```python
from build123d import *

# Parameters (mm, degrees)
F0_W     = 106.68
F0_H     = 157.48
F1_DEPTH = 106.68
F2_W     = 100.33
F2_H     = 151.13
F3_DEPTH = 101.6
F4_W     = 106.68
F4_H     = 1.5875
F5_DEPTH = 101.6
F6_R     = 5.08


with BuildPart() as f1:
    # F0 (on Front) → F1 (new body)
    with BuildSketch(Plane.XZ):
        with Locations((2.224307, 32.226964)):
            Rectangle(F0_W, F0_H)
    extrude(amount=F1_DEPTH)

    # F2 (on face) → F3 (cut)
    with BuildSketch(Plane.XZ.offset(106.68)):
        with Locations((2.224307, 32.226964)):
            Rectangle(F2_W, F2_H)
    extrude(amount=-F3_DEPTH, mode=Mode.SUBTRACT)

    # F4 (on face) → F5 (join)
    with BuildSketch(Plane.XZ.offset(106.68)):
        with Locations((2.224307, 56.198214)):
            Rectangle(F4_W, F4_H)
        with Locations((2.224307, 57.785714)):
            Rectangle(F4_W, F4_H)
        with Locations((2.224307, 6.985714)):
            Rectangle(F4_W, F4_H)
        with Locations((2.224307, 5.398214)):
            Rectangle(F4_W, F4_H)
    extrude(amount=-F5_DEPTH)

    # F6
    f6_edges = [f1.edges().sort_by_distance(p)[0] for p in [
        (55.564307, -53.34, 110.966964),
        (-51.115693, -53.34, 110.966964),
        (55.564307, -53.34, -46.513036),
        (-51.115693, -53.34, -46.513036),
        (-51.115693, 0, 32.226964),
        (2.224307, 0, 110.966964),
        (55.564307, 0, 32.226964),
        (2.224307, 0, -46.513036),
    ]]
    fillet(f6_edges, radius=F6_R)


solid = f1.part
```
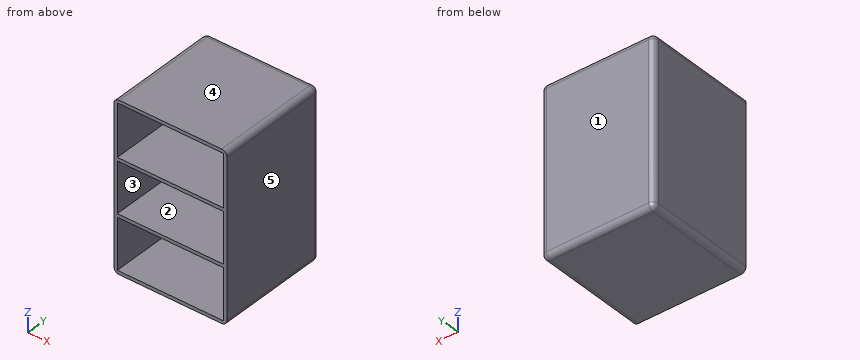
Here's how the part is built. I have some questions about the finished solid (model axes, mm). Face numbers are marked on the shaded views. A direction names the side the tool comes from. Round coordinates to 2 decimals unless told otherwise and drop trailing zeros. Order: outer loops, then holes, each group sorted by start corner. A loop starts at its lowest first (then second) coordinate and runs counter-clockwise, first axis right, second up. Notation, with made-up numbers: (-9.75, 44) -> (9.25, 44) arc R24 cw to (9.25, 78) -> close; hole circle Ø9 at (26.5, 30.5). An arc over 180 degrees is marked (long way). Use a Markdown table: item, result. Add a question column.
(1) Suppose I cut it at B-B, the plane y = -97. Please give me the cut outline in (x, z).
(2) Suppose I cut it at A-A, the plane z = 61. Please give me the cut outline in (x, y), and give its area (3 significant figures).
(3) For the marked faces 1 and 2, which set-ups out of +Z, -Z, +X, -X, +Y, -Y let a thin tool reach every point of the face, with its end or its side?
(4) For pin 1 Ø14.5 at (x, z) = (-16.5, 25) entering from -Y, with a flat end and sliding along its axis, tell me the tip position at first contact or that it passes through.
(5) Suppose I cut it at C-C, the plane x = -1. Please give me the cut outline in (y, z).
(6) If we mould it in two halves opening along X, with no side actions, what happens to the marked faces 3, 4 and 5? For each: released by +X, released by -X, zero draft, split by the parting line, or undercut.
(7) I need wall thicknesses on line 1 along Z through (x, y) = (38.5, -101); line 2 along X through (y, z) = (-80, 50); line 3 along Y through (x, z) = (-15, 89). Which ranges of each line are inside material? Lowest first, please.
Verdict:
| question | item | result |
|---|---|---|
| 1 | outline | (-51.12, -41.43) arc R5.08 ccw to (-46.04, -46.51) -> (50.48, -46.51) arc R5.08 ccw to (55.56, -41.43) -> (55.56, 105.89) arc R5.08 ccw to (50.48, 110.97) -> (-46.04, 110.97) arc R5.08 ccw to (-51.12, 105.89) -> close; hole (-47.94, -43.34) -> (52.39, -43.34) -> (52.39, 4.6) -> (-47.94, 4.6) -> close; hole (-47.94, 7.78) -> (52.39, 7.78) -> (52.39, 55.4) -> (-47.94, 55.4) -> close; hole (-47.94, 58.58) -> (52.39, 58.58) -> (52.39, 107.79) -> (-47.94, 107.79) -> close |
| 2 | outline | (-51.12, -106.68) -> (-47.94, -106.68) -> (-47.94, -5.08) -> (52.39, -5.08) -> (52.39, -106.68) -> (55.56, -106.68) -> (55.56, -5.08) arc R5.08 ccw to (50.48, 0) -> (-46.04, 0) arc R5.08 ccw to (-51.12, -5.08) -> close |
| 2 | area | 1,180 mm2 |
| 3 | face 1 | +Z, -Z, +X, -X, +Y |
| 3 | face 2 | -Y |
| 4 | pin 1 | y = -5.08 |
| 5 | outline | (-106.68, -46.51) -> (-5.08, -46.51) arc R5.08 ccw to (0, -41.43) -> (0, 105.89) arc R5.08 ccw to (-5.08, 110.97) -> (-106.68, 110.97) -> (-106.68, 107.79) -> (-5.08, 107.79) -> (-5.08, 58.58) -> (-106.68, 58.58) -> (-106.68, 55.4) -> (-5.08, 55.4) -> (-5.08, 7.78) -> (-106.68, 7.78) -> (-106.68, 4.6) -> (-5.08, 4.6) -> (-5.08, -43.34) -> (-106.68, -43.34) -> close |
| 6 | face 3 | undercut |
| 6 | face 4 | zero draft |
| 6 | face 5 | released by +X |
| 7 | line 1 | -46.51 to -43.34, 4.6 to 7.78, 55.4 to 58.58, 107.79 to 110.97 |
| 7 | line 2 | -51.12 to -47.94, 52.39 to 55.56 |
| 7 | line 3 | -5.08 to 0 |
